Answer from the drawing. Dimensions are ordinates in mm from the lowest x, y and z of the part. A direction names the side the tool comes from. Round coordinates to 2 decimals unless told otherwise and drop trailing zeros. Order: outer loops, then holes, each group sorted by start corner. A loop starts at its lowest first (then second) coordinate and runs counter-clockwise, first axis right, second up. Notation, with made-up numbers: M 48.5,0 L 103.5,0 A21 cw 103.5,22 Z; hole C 51,61.5 d4. An arc over 180 degrees is marked long. Write item = value, one per line. Start each with the question number.
(1) A cutting plane is placed at A-A, the plane x = 46.5. Determine the outline of the cut face in (y, z), and give its area (3 significant figures).
(2) A cutting plane is placed at C-C, the plane y = 9.5. Determine the outline of the cut face in (x, z).
(3) A cutting plane is placed at D-D, the plane z = 3.5. Determine the outline of the cut face in (x, y).
(4) Which of the six approach directions +Z, -Z, +X, -X, +Y, -Y give full straight-line access (tool end or side, diameter ignored) to the marked faces 1, 2, 3, 4 and 5?
(5) A cutting plane is placed at B-B, the plane z = 16. Determine the outline of the cut face in (x, y).
(6) Straight lines are drawn through the part: probe 1 along Y at (x, z) = (12.7, 11.85); probe 2 along X at (y, z) = (12.7, 20.5); probe 3 along Z at (x, y) = (10, 12.7). For each, find the intervals that lie inside material, in ascending order. Write a range as from..to.
(7) For a pull along Y with two mould halves and no side action, classify the marked faces 6, 7, 8 and 9 as released by +Y, released by -Y, zero draft, split by the parting line, or undercut.
(8) Each of these flat-tipped pins is pushed along its axis until it touches: pin 1 (8 mm diameter, centred on x = 15.5, z = 3, fed in from -Y); pin 2 (5 mm diameter, centred on x = 10.5, y = 18, fed in from -Z); pin 3 (4 mm diameter, centred on x = 25.4, y = 12.7, fed in from +Z); pin 4 (5 mm diameter, centred on y = 11, z = 12.5, fed in from -X). Where does it stop, or does it pass through?
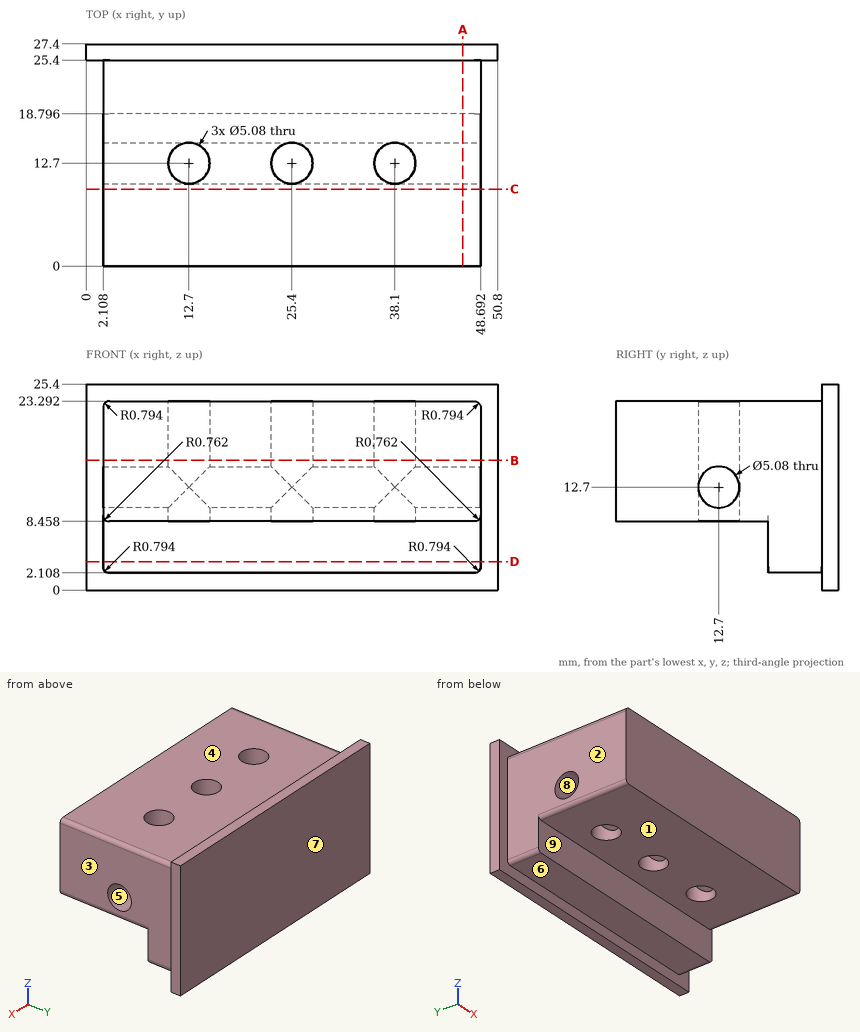
Reported:
q1.outline = M 0,8.46 L 18.8,8.46 L 18.8,2.11 L 25.4,2.11 L 25.4,0 L 27.4,0 L 27.4,25.4 L 25.4,25.4 L 25.4,23.29 L 0,23.29 Z; hole C 12.7,12.7 d5.08
q1.area = 449 mm²
q2.outline = M 2.11,9.22 A0.76 ccw 2.87,8.46 L 47.93,8.46 A0.76 ccw 48.69,9.22 L 48.69,22.5 A0.79 ccw 47.9,23.29 L 2.9,23.29 A0.79 ccw 2.11,22.5 Z
q3.outline = M 0,25.4 L 2.11,25.4 L 2.11,18.8 L 48.69,18.8 L 48.69,25.4 L 50.8,25.4 L 50.8,27.4 L 0,27.4 Z
q4.face_1 = -Z, +X, -X, -Y
q4.face_2 = +Z, -Z, -X, -Y
q4.face_3 = +Z, -Z, +X, -Y
q4.face_4 = +Z, +X, -X, -Y
q4.face_5 = +X, -X
q5.outline = M 0,25.4 L 2.11,25.4 L 2.11,0 L 48.69,0 L 48.69,25.4 L 50.8,25.4 L 50.8,27.4 L 0,27.4 Z; hole C 12.7,12.7 d5.08; hole C 25.4,12.7 d5.08; hole C 38.1,12.7 d5.08
q6.probe_1 = 0..10.16, 15.24..27.4
q6.probe_2 = 2.11..10.16, 15.24..22.86, 27.94..35.56, 40.64..48.69
q6.probe_3 = 8.46..10.16, 15.24..23.29
q7.face_6 = zero draft
q7.face_7 = released by +Y
q7.face_8 = undercut
q7.face_9 = released by -Y
q8.pin_1 = 18.8
q8.pin_2 = 2.11
q8.pin_3 = through
q8.pin_4 = 2.11
